from build123d import *

# Parameters (mm, degrees)
SKETCH1_W           = 150
SKETCH1_H           = 150
BOSS_EXTRUDE1_DEPTH = 3.5
SKETCH2_W           = 142.8
SKETCH2_H           = 142.8
BOSS_EXTRUDE2_DEPTH = 3.5
FILLET9_R           = 10
FILLET10_R          = 10
CHAMFER3_SIZE       = 3
SKETCH3_W           = 10
SKETCH3_H           = 5
CUT_EXTRUDE1_DEPTH  = 10
SKETCH4_W           = 10
SKETCH4_H           = 5
CUT_EXTRUDE2_DEPTH  = 10
SKETCH5_W           = 10
SKETCH5_H           = 5
CUT_EXTRUDE3_DEPTH  = 10
SKETCH6_W           = 10
SKETCH6_H           = 5
CUT_EXTRUDE4_DEPTH  = 10


with BuildPart() as part:
    # Sketch1 → Boss-Extrude1 (new body)
    with BuildSketch(Plane(origin=(0, 0, 0), x_dir=(1, 0, 0), z_dir=(0, 1, 0))):
        with Locations((75, 75)):
            Rectangle(SKETCH1_W, SKETCH1_H)
    extrude(amount=BOSS_EXTRUDE1_DEPTH)

    # Sketch2 → Boss-Extrude2 (add)
    with BuildSketch(Plane(origin=(0, 3.5, 0), x_dir=(1, 0, 0), z_dir=(0, 1, 0))):
        with Locations((75, 75)):
            Rectangle(SKETCH2_W, SKETCH2_H)
    extrude(amount=BOSS_EXTRUDE2_DEPTH)

    # Fillet9
    fillet9_edges = [part.edges().sort_by_distance(p)[0] for p in [
        (146.4, 5.25, -3.6),
        (150, 1.75, 0),
    ]]
    fillet(fillet9_edges, radius=FILLET9_R)

    # Fillet10
    fillet10_edges = [part.edges().sort_by_distance(p)[0] for p in [
        (3.6, 5.25, -146.4),
        (3.6, 5.25, -3.6),
        (146.4, 5.25, -146.4),
        (0, 1.75, -150),
        (150, 1.75, -150),
        (0, 1.75, 0),
    ]]
    fillet(fillet10_edges, radius=FILLET10_R)

    # Chamfer3
    chamfer3_edges = [part.edges().sort_by_distance(p)[0] for p in [
        (150, 0, -75),
        (147.071067812, 0, -2.928932188),
        (0, 0, -75),
        (75, 0, 0),
        (75, 0, -150),
        (147.071067812, 0, -147.071067812),
        (2.928932188, 0, -2.928932188),
        (2.928932188, 0, -147.071067812),
    ]]
    chamfer(chamfer3_edges, length=CHAMFER3_SIZE)

    # Sketch3 → Cut-Extrude1 (cut)
    with BuildSketch(Plane(origin=(0, 7, 0), x_dir=(1, 0, 0), z_dir=(0, 1, 0))):
        with Locations((22, 19.5)):
            Rectangle(SKETCH3_W, SKETCH3_H)
    extrude(amount=-CUT_EXTRUDE1_DEPTH, mode=Mode.SUBTRACT)

    # Sketch4 → Cut-Extrude2 (cut)
    with BuildSketch(Plane(origin=(0, 7, 0), x_dir=(1, 0, 0), z_dir=(0, 1, 0))):
        with Locations((22, 130.5)):
            Rectangle(SKETCH4_W, SKETCH4_H)
    extrude(amount=-CUT_EXTRUDE2_DEPTH, mode=Mode.SUBTRACT)

    # Sketch5 → Cut-Extrude3 (cut)
    with BuildSketch(Plane(origin=(0, 7, 0), x_dir=(1, 0, 0), z_dir=(0, 1, 0))):
        with Locations((128, 19.5)):
            Rectangle(SKETCH5_W, SKETCH5_H)
    extrude(amount=-CUT_EXTRUDE3_DEPTH, mode=Mode.SUBTRACT)

    # Sketch6 → Cut-Extrude4 (cut)
    with BuildSketch(Plane(origin=(0, 7, 0), x_dir=(1, 0, 0), z_dir=(0, 1, 0))):
        with Locations((128, 130.5)):
            Rectangle(SKETCH6_W, SKETCH6_H)
    extrude(amount=-CUT_EXTRUDE4_DEPTH, mode=Mode.SUBTRACT)


solid = part.part
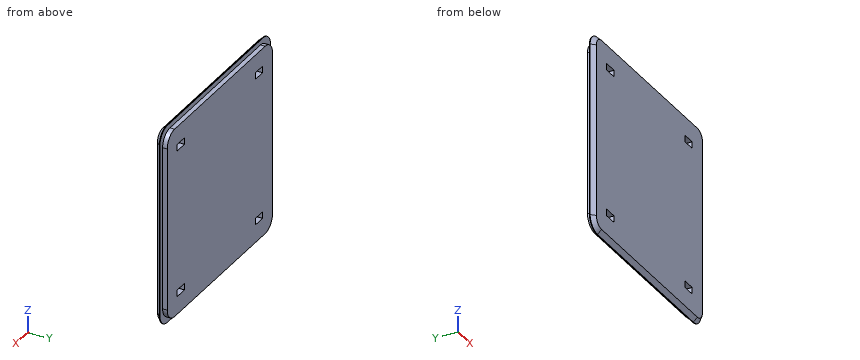
For this review, take the finished solid that the model builds, in its own axes (mm). Coordinates: 2 decimals unless noted, no trailing zeros. Write each loop counter-clockwise with the first axis right and the second up, starting at its lowest first coordinate (ties: lowest second). Pieces come first, ordered by that corner, then holes. Notation, with made-up numbers: (28.25, 5.5) -> (63.25, 5.5) arc R23 cw to (63.25, 14.5) -> close; hole circle Ø5 at (-10, 69). An arc over 180 degrees is marked (long way). Write each question's results on one line, items separated by ' | '. Start each with the question number.
1) Insertion check: pin 1 (1.5 mm diameter, centred on y = 4.5, z = -130.5, fed in from -X); pin 2 (1.8 mm diameter, centred on y = 4.5, z = -92.5, fed in from +X). Each pin has a flat end and moves straight along its axis. Give the tip position at first contact, or say it passes through.
2) Consider section B-B (x = 56). Write out the cut boundary in (y, z).
3) Consider section A-A (z = -95). Write out the cut boundary in (x, y), plus the area to 3 significant figures.
4) Wall thickness on L1, parallel to Z at x = 17.5, y = 3.25; L2, parallel to Z at x = 69.5, y = 5.75; L3, parallel to X at y = 6.25, z = -47.5: over which ranges is each line inside the solid? List them lowest first. Write a range as [from, to].
Geometry says:
1) pin 1: x = 3.6 | pin 2: x = 146.4
2) outline: (0, -147) -> (3, -150) -> (3.5, -150) -> (3.5, -146.4) -> (7, -146.4) -> (7, -3.6) -> (3.5, -3.6) -> (3.5, 0) -> (3, 0) -> (0, -3) -> close
3) outline: (0, 3) -> (3, 0) -> (147, 0) -> (150, 3) -> (150, 3.5) -> (146.4, 3.5) -> (146.4, 7) -> (3.6, 7) -> (3.6, 3.5) -> (0, 3.5) -> close | area: 1,020 mm^2
4) L1: [-150, -133], [-128, -22], [-17, 0] | L2: [-146.4, -3.6] | L3: [3.6, 146.4]
